from build123d import *

# Parameters (mm, degrees)
BOSS_EXTRUDE3_DEPTH      = 51
BOSS_EXTRUDE3_DEPTH_BACK = 51
CUT_EXTRUDE3_REACH       = 179.381
SKETCH7_R                = 1.5635
SKETCH7_R_2              = 28.5
CUT_EXTRUDE4_REACH       = 278.066
SKETCH8_R                = 14.2875


with BuildPart() as part:
    # Sketch6 → Boss-Extrude3 (new, two sides: drawn at the far end of the back side and taken through both)
    with BuildSketch(Plane(origin=(0, 0, 0), x_dir=(1, 0, 0), z_dir=(0, 1, 0)).offset(-BOSS_EXTRUDE3_DEPTH_BACK)):
        Polygon((183.723, -47.5), (183.723, -54.5), (64.5, -54.5), (64.5, 88.773061806), (-64.5, 88.773061806), (-64.5, -48.5), (-70.5, -48.5), (-70.5, 94.773061806), (70.5, 94.773061806), (70.5, -47.5), align=None)
    extrude(amount=BOSS_EXTRUDE3_DEPTH + BOSS_EXTRUDE3_DEPTH_BACK)

    # Sketch7 → Cut-Extrude3 (cut, up to next)
    with BuildSketch(Plane(origin=(70.5, 0, 0), x_dir=(0, 0, -1), z_dir=(1, 0, 0)), mode=Mode.PRIVATE) as cut_extrude3_sk1:
        with Locations((0, 42.5)):
            Circle(SKETCH7_R)
    cut_extrude3_tool1 = extrude(cut_extrude3_sk1.sketch, amount=-CUT_EXTRUDE3_REACH, mode=Mode.PRIVATE) & part.part
    # Sketch7 → Cut-Extrude3 (cut, up to next)
    with BuildSketch(Plane(origin=(70.5, 0, 0), x_dir=(0, 0, -1), z_dir=(1, 0, 0)), mode=Mode.PRIVATE) as cut_extrude3_sk2:
        with Locations((42.5, 0)):
            Circle(SKETCH7_R)
    cut_extrude3_tool2 = extrude(cut_extrude3_sk2.sketch, amount=-CUT_EXTRUDE3_REACH, mode=Mode.PRIVATE) & part.part
    # Sketch7 → Cut-Extrude3 (cut, up to next)
    with BuildSketch(Plane(origin=(70.5, 0, 0), x_dir=(0, 0, -1), z_dir=(1, 0, 0)), mode=Mode.PRIVATE) as cut_extrude3_sk3:
        with Locations((0, -42.5)):
            Circle(SKETCH7_R)
    cut_extrude3_tool3 = extrude(cut_extrude3_sk3.sketch, amount=-CUT_EXTRUDE3_REACH, mode=Mode.PRIVATE) & part.part
    # Sketch7 → Cut-Extrude3 (cut, up to next)
    with BuildSketch(Plane(origin=(70.5, 0, 0), x_dir=(0, 0, -1), z_dir=(1, 0, 0)), mode=Mode.PRIVATE) as cut_extrude3_sk4:
        with Locations((-42.5, 0)):
            Circle(SKETCH7_R)
    cut_extrude3_tool4 = extrude(cut_extrude3_sk4.sketch, amount=-CUT_EXTRUDE3_REACH, mode=Mode.PRIVATE) & part.part
    # Sketch7 → Cut-Extrude3 (cut, up to next)
    with BuildSketch(Plane(origin=(70.5, 0, 0), x_dir=(0, 0, -1), z_dir=(1, 0, 0)), mode=Mode.PRIVATE) as cut_extrude3_sk5:
        Circle(SKETCH7_R_2)
    cut_extrude3_tool5 = extrude(cut_extrude3_sk5.sketch, amount=-CUT_EXTRUDE3_REACH, mode=Mode.PRIVATE) & part.part
    add(cut_extrude3_tool1.solids().sort_by_distance((70.5, 42.5, 0))[0], mode=Mode.SUBTRACT)
    add(cut_extrude3_tool2.solids().sort_by_distance((70.5, 0, -42.5))[0], mode=Mode.SUBTRACT)
    add(cut_extrude3_tool3.solids().sort_by_distance((70.5, -42.5, 0))[0], mode=Mode.SUBTRACT)
    add(cut_extrude3_tool4.solids().sort_by_distance((70.5, 0, 42.5))[0], mode=Mode.SUBTRACT)
    add(cut_extrude3_tool5.solids().sort_by_distance((70.5, 0, 0))[0], mode=Mode.SUBTRACT)

    # Sketch8 → Cut-Extrude4 (cut, up to next)
    with BuildSketch(Plane.ZY.offset(70.5), mode=Mode.PRIVATE) as cut_extrude4_sk1:
        Circle(SKETCH8_R)
    cut_extrude4_tool1 = extrude(cut_extrude4_sk1.sketch, amount=-CUT_EXTRUDE4_REACH, mode=Mode.PRIVATE) & part.part
    add(cut_extrude4_tool1.solids().sort_by_distance((-70.5, 0, 0))[0], mode=Mode.SUBTRACT)


solid = part.part
Design review of the part built by this model. Coordinates are the model's own, in mm. A direction names the side the tool comes from. Give positions to 0.01 mm unless a question says otherwise; leave off trailing zeros. Write each loop counter-clockwise with the first axis right and the second up, starting at its lowest first coordinate (ties: lowest second). Pieces come first, ordered by that corner, then holes. Notation, with made-up numbers: M -18,35 L 31,35 A14 cw 31,39 Z; hole C -33.5,0 d11. An arc over 180 degrees is marked long. Answer as a JSON object with one key per item and string values. Group by question number.
1) We need section D-D (x = 47). Give the boundary of the cut face in (y, z), and give its area (3 significant figures).
2) Tool access review of faces 4 (the face through (-64.5, -1, -21)), 5 (the face through (-67.542, 0.628, -14.274)), 6 (the face through (-67, -1, 48.5)), 7 (the face through (-70.5, -1, -22)), 8 (the face through (126, -1, 47.5)): name each direction out of +Z, -Z, +X, -X, +Y, -Y from which nothing blocks a thin tool from reaching the whole face with its end or side.
3) We need section A-A (z = 38). Give the boundary of the cut face in (x, y).
4) We need section C-C (x = 142). Give the boundary of the cut face in (y, z).
5) Clearance check with flat-ended pins moving along their axes: pin 1 Ø23 at (y, z) = (0, 0) entering from -X; pin 2 Ø1 at (y, z) = (11.5, -14.5) entering from +X; pin 3 Ø3 at (x, y) = (-13, 4) entering from +Z; pin 4 Ø5 at (x, y) = (-68, -8) entering from +Z. State where each tip first meets the part, or that it passes through.
6) We need section B-B (z = -20). Give the boundary of the cut face in (x, y), and give its area (3 significant figures).
7) For line 1 along Y through (x, z) = (68, 0); line 2 along X through (y, z) = (-11, 26.5); line 3 along Y through (x, z) = (67.7, 42.5), list the stretches that pass through material, from the lowest coordinate up.
8) Mouldability with a two-part tool opening along Y and no side actions: class faces 1 (the face through (64.5, -1, -32)), 2 (the face through (67, 51, -20)), 3 (the face through (67.542, -10.916, -26.327)) as released by +Y, released by -Y, zero draft, split by the parting line, or undercut.
Answer key:
{
 "1": {"outline": "M -51,-94.77 L 51,-94.77 L 51,-88.77 L -51,-88.77 Z", "area": "612 mm²"},
 "2": {"face 4": "+Z, +Y, -Y", "face 5": "+X, -X", "face 6": "+Z, -X, +Y, -Y", "face 7": "+Z, -Z, -X, +Y, -Y", "face 8": "-Z, +X, +Y, -Y"},
 "3": {"outline": "M -70.5,-51 L -64.5,-51 L -64.5,51 L -70.5,51 Z; M 64.5,-51 L 70.5,-51 L 70.5,51 L 64.5,51 Z"},
 "4": {"outline": "M -51,47.5 L 51,47.5 L 51,54.5 L -51,54.5 Z"},
 "5": {"pin 1": "passes through", "pin 2": "stops at x = -64.5", "pin 3": "stops at z = -88.77", "pin 4": "stops at z = 48.5"},
 "6": {"outline": "M -70.5,-51 L -64.5,-51 L -64.5,51 L -70.5,51 Z; M 64.5,-51 L 70.5,-51 L 70.5,-20.3 L 64.5,-20.3 Z; M 64.5,20.3 L 70.5,20.3 L 70.5,51 L 64.5,51 Z", "area": "980 mm²"},
 "7": {"line 1": "y = -51 to -44.06, -40.94 to -28.5, 28.5 to 40.94, 44.06 to 51", "line 2": "x = -70.5 to -64.5, 64.5 to 70.5", "line 3": "y = -51 to -1.56, 1.56 to 51"},
 "8": {"face 1": "zero draft", "face 2": "released by +Y", "face 3": "undercut"}
}
